The model under review builds one solid part; all positions refer to its coordinate system, in mm. Round coordinates to 2 decimals unless told otherwise and drop trailing zeros. Write each loop counter-clockwise with the first axis right and the second up, starting at its lowest first coordinate (ties: lowest second). Pieces come first, ordered by that corner, then holes. Notation, with made-up numbers: M 11,-40 L 20,-40 A20 ccw 20,-16 Z; hole C 45.25,15.25 d8. An arc over 180 degrees is marked long. Write item = value, one per line. Start each with the question number.
Item 1: Take a section at B-B, the plane x = -111. Give the boundary of the cut face in (y, z).
Item 2: Take a section at A-A, the plane y = 111. Give the boundary of the cut face in (x, z), plus the area to 3 significant figures.
Item 3: Take a section at C-C, the plane z = 327.5. Give the boundary of the cut face in (x, y), plus the area to 3 significant figures.
Item 4: For pin 1 Ø1.5 at (x, z) = (-107, 421.5) entering from +Y; pin 2 Ø5 at (y, z) = (110.5, 325.5) entering from -X; pin 3 Ø10 at (x, z) = (-112.5, 395.5) entering from +Y, all flat-tipped, find the tip position at first contact; note any pin that passes through.
Item 5: To check wall thickness, follow line 1 along X through (y, z) = (110.5, 463.5); line 2 along Y through (x, z) = (-110.75, 354); line 3 along X through (y, z) = (111.75, 473.5). State the ranges of each line that lie inside material, in increasing order.
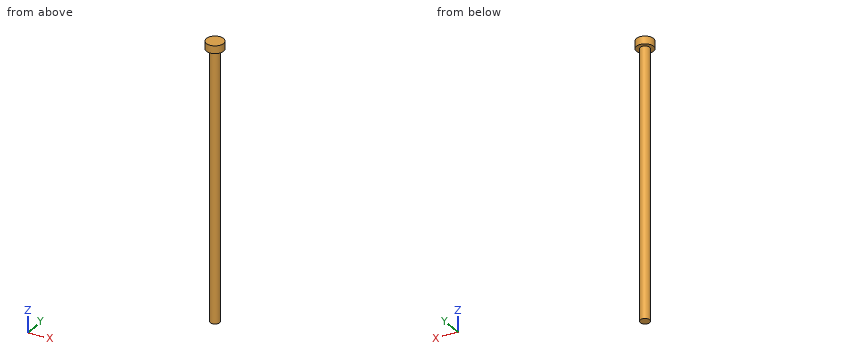
from build123d import *

# Parameters (mm, degrees)
EXTRUDE_START      = 225
EXTRUDE_SKETCH_1_R = 5
EXTRUDE_1_DEPTH    = 280
EXTRUDE_START_2    = 505
EXTRUDE_SKETCH_2_R = 9
EXTRUDE_2_DEPTH    = 8


with BuildPart() as part:
    # Extrude sketch 1 → Extrude 1 (new body)
    with BuildSketch(Plane.XY.offset(EXTRUDE_START)):
        with Locations((-111, 111)):
            Circle(EXTRUDE_SKETCH_1_R)
    extrude(amount=EXTRUDE_1_DEPTH)


with BuildPart() as body_2:
    # Extrude sketch 2 → Extrude 2 (new body)
    with BuildSketch(Plane.XY.offset(EXTRUDE_START_2)):
        with Locations((-111, 111)):
            Circle(EXTRUDE_SKETCH_2_R)
    extrude(amount=EXTRUDE_2_DEPTH)

    # Combine (weld / assembly of features): union part
    add(part.part)


solid = body_2.part
Response values:
q1.outline = M 102,505 L 106,505 L 106,225 L 116,225 L 116,505 L 120,505 L 120,513 L 102,513 Z
q2.outline = M -120,505 L -116,505 L -116,225 L -106,225 L -106,505 L -102,505 L -102,513 L -120,513 Z
q2.area = 2,940 mm2
q3.outline = C -111,111 d10
q3.area = 78.5 mm2
q4.pin_1 = 114.8
q4.pin_2 = -116
q4.pin_3 = 116
q5.line_1 = -115.97 to -106.03
q5.line_2 = 106.01 to 115.99
q5.line_3 = -115.94 to -106.06
